Could you check a few things on this drawing? It's one solid part, dimensions in mm from its lowest x, y, z. A direction names the side the tool comes from. Coordinates: 2 decimals unless noted, no trailing zeros. Loops run counter-clockwise (first coordinate to the right, second up) from the corner with the lowest first, then second, coordinate; pieces in that order, holes last.
1) Imagine slicing it at A-A on x = 7.25. Please give me the cut outline in (y, z), plus the area to 4 significant figures.
2) If I drill on line 1 along X through (y, z) = (7, 1.3); line 2 along X through (y, z) = (3.75, 1.35); line 3 along Y through (x, z) = (4.5, 1.2), over which ranges is the centre line in solid material (lowest first)?
3) Imagine slicing it at C-C on z = 0.8. Please give me the cut outline in (x, y).
4) Will these pins go through, and if not, where does the flat tip stop? P1, Ø4, axis at x = 6.5, y = 7, coming from the -Z side; P2, Ø1, axis at y = 4, z = 0.5, coming from the +X side.
5) For the marked faces 4 and 5, which set-ups out of +Z, -Z, +X, -X, +Y, -Y let a thin tool reach every point of the face, with its end or its side?
6) Imagine slicing it at B-B on y = 7.25. Please give me the cut outline in (x, z).
7) Thinking about a two-plate mould opening in X: for the marked faces 1, 2 and 3, which applies, released by +X, released by -X, zero draft, split by the parting line, or undercut?
8) Imagine slicing it at D-D on y = 2. Please give me the cut outline in (x, z), plus the area to 3 significant figures.
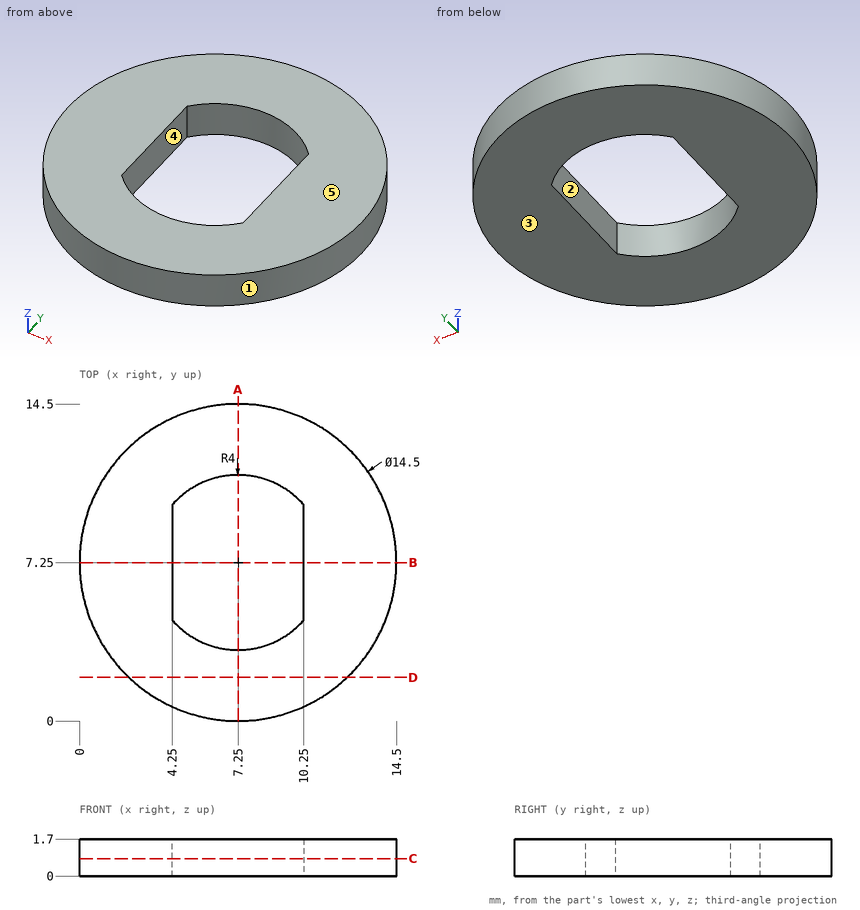
Filled in:
1. outline: (0, 0) - (3.25, 0) - (3.25, 1.7) - (0, 1.7) - close; (11.25, 0) - (14.5, 0) - (14.5, 1.7) - (11.25, 1.7) - close
1. area: 11.05 mm2
2. line 1: x = 0 to 4.25, 10.25 to 14.5
2. line 2: x = 0.9 to 5.31, 9.19 to 13.6
2. line 3: y = 0.54 to 4.35, 10.15 to 13.96
3. outline: circle Ø14.5 at (7.25, 7.25); hole (4.25, 4.6) arc R4 ccw to (10.25, 4.6) - (10.25, 9.9) arc R4 ccw to (4.25, 9.9) - close
4. P1: passes through
4. P2: stops at x = 13.96
5. face 4: +Z, -Z
5. face 5: +Z, +X, -X, +Y, -Y
6. outline: (0, 0) - (4.25, 0) - (4.25, 1.7) - (0, 1.7) - close; (10.25, 0) - (14.5, 0) - (14.5, 1.7) - (10.25, 1.7) - close
7. face 1: split by the parting line
7. face 2: undercut
7. face 3: zero draft
8. outline: (2.25, 0) - (12.25, 0) - (12.25, 1.7) - (2.25, 1.7) - close
8. area: 17.0 mm2
